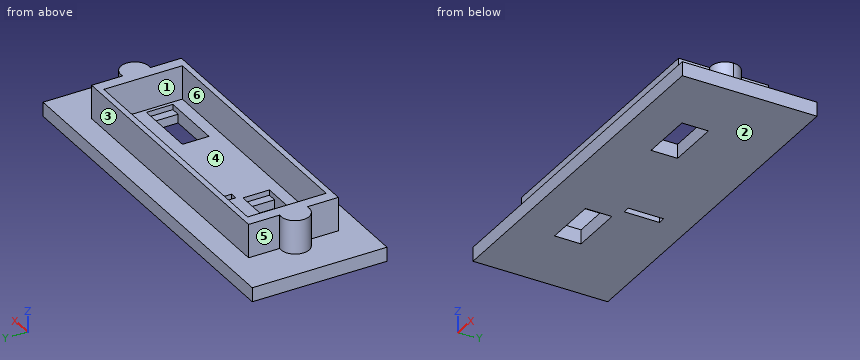
from build123d import *

# Parameters (mm, degrees)
F0_W     = 203.2
F0_H     = 76.2
F1_DEPTH = 8
F2_W     = 152.4
F2_H     = 50.8
F2_W_2   = 139.7
F2_H_2   = 44.45
F4_DEPTH = 19.05
F5_W     = 30
F5_H     = 15
F6_DEPTH = 8
F5_W_2   = 4
F5_H_2   = 20
F7_DEPTH = 8
F8_W     = 5
F8_H     = 15
F9_DEPTH = 3


with BuildPart() as f1:
    # F0 (on Top) → F1 (new body)
    with BuildSketch(Plane.XY):
        Rectangle(F0_W, F0_H)
    extrude(amount=F1_DEPTH)

    # F2 (on face) + F3 (on face) → F4 (join)
    with BuildSketch(Plane.XY.offset(8)):
        Rectangle(F2_W, F2_H)
        Rectangle(F2_W_2, F2_H_2, mode=Mode.SUBTRACT)
    with BuildSketch(Plane.XY.offset(8)):
        with BuildLine():
            Line((-76.2, -7.7771299333), (-76.2, 7.7771299333))
            ThreePointArc((-76.2, 7.7771299333), (-85.725, 0), (-76.2, -7.7771299333))
        make_face()
        with BuildLine():
            ThreePointArc((85.725, 0), (82.8076157855, 6.1483610621), (76.2, 7.7771299333))
            Line((76.2, 7.7771299333), (76.2, -7.7771299333))
            ThreePointArc((76.2, -7.7771299333), (82.8076157855, -6.1483610621), (85.725, 0))
        make_face()
    extrude(amount=F4_DEPTH)

    # F5 (on face) → F6 (cut, through all)
    with BuildSketch(Plane.XY.offset(8)):
        with Locations((47.85, -8.225)):
            Rectangle(F5_W, F5_H)
        with Locations((-45.85, -8.225)):
            Rectangle(F5_W, F5_H)
    extrude(amount=-F6_DEPTH, mode=Mode.SUBTRACT)

    # F5 (on face) → F7 (cut, through all)
    with BuildSketch(Plane.XY.offset(8)):
        with Locations((-22, 12.225)):
            Rectangle(F5_W_2, F5_H_2)
    extrude(amount=-F7_DEPTH, mode=Mode.SUBTRACT)

    # F8 (on face) → F9 (cut)
    with BuildSketch(Plane.XY.offset(8)):
        with Locations((65.35, -8.225)):
            Rectangle(F8_W, F8_H)
        with Locations((-28.35, -8.225)):
            Rectangle(F8_W, F8_H)
    extrude(amount=-F9_DEPTH, mode=Mode.SUBTRACT)


solid = f1.part
The listing builds one solid part. Answer for the finished solid, in the listing's coordinates (mm). Face numbers are marked on the shaded views. A direction names the side the tool comes from. Give positions to 0.01 mm unless a question says otherwise; leave off trailing zeros. Write each loop counter-clockwise with the first axis right and the second up, starting at its lowest first coordinate (ties: lowest second). Pieces come first, ordered by that corner, then holes. Notation, with made-up numbers: (76, -9) - (135, -9) arc R21 cw to (135, 22) - close; hole circle Ø5 at (35.25, 26). An arc over 180 degrees is marked (long way). Use a Markdown table: item, result.
1. Section C-C on y = 4 is taken. Write down the section's boundary in (x, z), plus the area to 3 significant figures.
Values follow:
| item | result |
|---|---|
| outline | (-101.6, 0) - (-24, 0) - (-24, 8) - (-69.85, 8) - (-69.85, 27.05) - (-84.64, 27.05) - (-84.64, 8) - (-101.6, 8) - close; (-20, 0) - (101.6, 0) - (101.6, 8) - (84.64, 8) - (84.64, 27.05) - (69.85, 27.05) - (69.85, 8) - (-20, 8) - close |
| area | 2,160 mm² |
2. Section B-B on z = 2 is taken. Write down the section's boundary in (x, y) (3 decimals), plus the area to 3 significant figures.
Values follow:
| item | result |
|---|---|
| outline | (-101.6, -38.1) - (101.6, -38.1) - (101.6, 38.1) - (-101.6, 38.1) - close; hole (-60.85, -15.725) - (-30.85, -15.725) - (-30.85, -0.725) - (-60.85, -0.725) - close; hole (-24, 2.225) - (-20, 2.225) - (-20, 22.225) - (-24, 22.225) - close; hole (32.85, -15.725) - (62.85, -15.725) - (62.85, -0.725) - (32.85, -0.725) - close |
| area | 14,500 mm² |
3. Each of these flat-tipped pins is pushed along its axis until it touches: P1, Ø1, axis at x = -77.5, z = 12.5, coming from the -Y side; P2, Ø4, axis at x = 64.5, y = -8, coming from the +Z side; P3, Ø12, axis at x = 8.5, z = 17.5, coming from the -Y side. Where does it stop, or does it pass through?
Values follow:
| item | result |
|---|---|
| P1 | stops at y = -7.94 |
| P2 | stops at z = 5 |
| P3 | stops at y = -25.4 |
4. A tool of negligible diameter and unlimited length cuts with its end or side. For the marked faces 1 and 2, from which of +Z, -Z, +X, -X, +Y, -Y can it reach the whole face along a straight path? Write none if from no direction.
Values follow:
| item | result |
|---|---|
| face 1 | +Z |
| face 2 | -Z, +X, -X, +Y, -Y |
5. For a pull along Y with two mould halves and no side action, classify the marked faces 3, 4, 5 and 6 as released by +Y, released by -Y, zero draft, split by the parting line, or undercut.
Values follow:
| item | result |
|---|---|
| face 3 | released by +Y |
| face 4 | undercut |
| face 5 | zero draft |
| face 6 | undercut |
6. Section A-A on x = -40.5 is taken. Write down the section's boundary in (y, z) (3 decimals), plus the area to 3 significant figures.
Values follow:
| item | result |
|---|---|
| outline | (-38.1, 0) - (-15.725, 0) - (-15.725, 8) - (-22.225, 8) - (-22.225, 27.05) - (-25.4, 27.05) - (-25.4, 8) - (-38.1, 8) - close; (-0.725, 0) - (38.1, 0) - (38.1, 8) - (25.4, 8) - (25.4, 27.05) - (22.225, 27.05) - (22.225, 8) - (-0.725, 8) - close |
| area | 611 mm² |
7. Section D-D on x = -5.5 is taken. Write down the section's boundary in (y, z) (3 decimals), plus the area to 3 significant figures.
Values follow:
| item | result |
|---|---|
| outline | (-38.1, 0) - (38.1, 0) - (38.1, 8) - (25.4, 8) - (25.4, 27.05) - (22.225, 27.05) - (22.225, 8) - (-22.225, 8) - (-22.225, 27.05) - (-25.4, 27.05) - (-25.4, 8) - (-38.1, 8) - close |
| area | 731 mm² |
8. Find the intervals of material crossed by probe 1 along X at (y, z) = (20.5, 10); probe 2 along Y at (x, z) = (6, 10.5) (3 decimals); probe 3 along X at (y, z) = (21, 7.75), in increasing order. Write a range as from..to.
Values follow:
| item | result |
|---|---|
| probe 1 | x = -76.2..-69.85, 69.85..76.2 |
| probe 2 | y = -25.4..-22.225, 22.225..25.4 |
| probe 3 | x = -101.6..-24, -20..101.6 |
